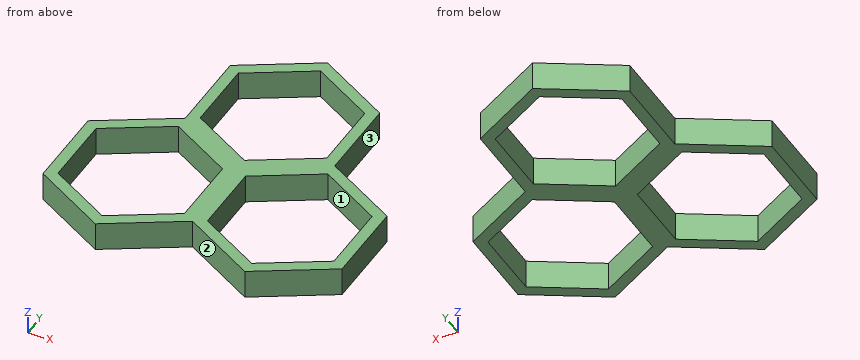
```python
from build123d import *

# Parameters (mm, degrees)
F1_DEPTH = 6.35
F2_T     = -2.54
F3_COUNT = 3
F3_ANGLE = 240


with BuildPart() as f1:
    # F0 (on Top) → F1 (new body)
    with BuildSketch(Plane.XY):
        Polygon((16.51, 9.5320529443), (0, 19.0641058886), (-16.51, 9.5320529443), (-16.51, -9.5320529443), (0, -19.0641058886), (16.51, -9.5320529443), align=None)
    extrude(amount=F1_DEPTH)

    # F2
    f2_openings = [f1.faces().sort_by_distance(p)[0] for p in [
        (0, 0, 6.35),
        (0, 0, 0),
    ]]
    offset(amount=F2_T, openings=f2_openings)

    # F3: F1 ×3 about axis
    f3_axis = Axis((0, -19.0641058886, 3.175), (0, 0, -1))


with BuildPart() as f1_1:
    add(f1.part)
    for i in range(1, F3_COUNT):
        add(f1.part.rotate(f3_axis, i * F3_ANGLE / (F3_COUNT - 1)))


solid = f1_1.part
```
The listing builds one solid part. Answer for the finished solid, in the listing's coordinates (mm). Face numbers are marked on the shaded views. A direction names the side the tool comes from. Coordinates: 2 decimals unless noted, no trailing zeros. Write each loop counter-clockwise with the first axis right and the second up, starting at its lowest first coordinate (ties: lowest second). Pieces come first, ordered by that corner, then holes. Notation, with made-up numbers: (29, 35) - (41, 35) arc R27 ccw to (41, 57) - close; hole circle Ø7 at (14, 23). An arc over 180 degrees is marked (long way). One line per item, written item: value.
1) Find section C-C (z = 2). Count the separate pieces of the cut face and the enclosed holes in it, and give its area (3 significant figures).
Geometry check:
separate pieces: 1
enclosed holes: 3
area: 805 mm2
2) A tool of negligible diameter and unlimited length cuts with its end or side. For the marked faces 1, 2 and 3, from which of +Z, -Z, +X, -X, +Y, -Y can it reach the whole face along a straight path? Write none if from no direction.
Geometry check:
face 1: +Z, -Z
face 2: +Z, -Z, -Y
face 3: +Z, -Z, +X, +Y
3) Find section A-A (y = -24). Give the vertices of the cut face in (x, z), and give its area (3 significant figures).
Geometry check:
outline: (-33.02, 0) - (-30.48, 0) - (-30.48, 6.35) - (-33.02, 6.35) - close; (-2.54, 0) - (2.54, 0) - (2.54, 6.35) - (-2.54, 6.35) - close; (30.48, 0) - (33.02, 0) - (33.02, 6.35) - (30.48, 6.35) - close
area: 64.5 mm2
4) Find section D-D (y = -5.5). Give the vertices of the cut face in (x, z), and give its area (3 significant figures).
Geometry check:
outline: (-16.51, 0) - (-13.97, 0) - (-13.97, 6.35) - (-16.51, 6.35) - close; (13.97, 0) - (16.51, 0) - (16.51, 6.35) - (13.97, 6.35) - close
area: 32.3 mm2
5) Each of these flat-tipped pins is pushed along its axis until it touches: pin 1 Ø2 at (x, z) = (-4, 2.5) entering from +Y; pin 2 Ø3 at (y, z) = (3, 1.5) entering from -X; pin 3 Ø1.9 at (y, z) = (-0.5, 5) entering from +X. Where does it stop, or does it pass through?
Geometry check:
pin 1: stops at y = 17.33
pin 2: stops at x = -16.51
pin 3: stops at x = 16.51
6) Find section B-B (x = -27.5). Give the vertices of the cut face in (y, z), and give its area (3 significant figures).
Geometry check:
outline: (-41.32, 0) - (-38.38, 0) - (-38.38, 6.35) - (-41.32, 6.35) - close; (-18.81, 0) - (-15.88, 0) - (-15.88, 6.35) - (-18.81, 6.35) - close
area: 37.2 mm2
7) Consider line 1 along X through (y, z) = (-34, 5); line 2 along Y through (x, z) = (9, 5.5); line 3 along Y through (x, z) = (-5, 5.25). Determine where each line is inside the solid, lowest interval first. Write a range as from..to.
Geometry check:
line 1: x = -33.02..-30.48, -2.54..2.54, 30.48..33.02
line 2: y = -43.32..-40.39, -16.8..-10.94, 10.94..13.87
line 3: y = -41.01..-38.08, -19.11..-13.24, 13.24..16.18
